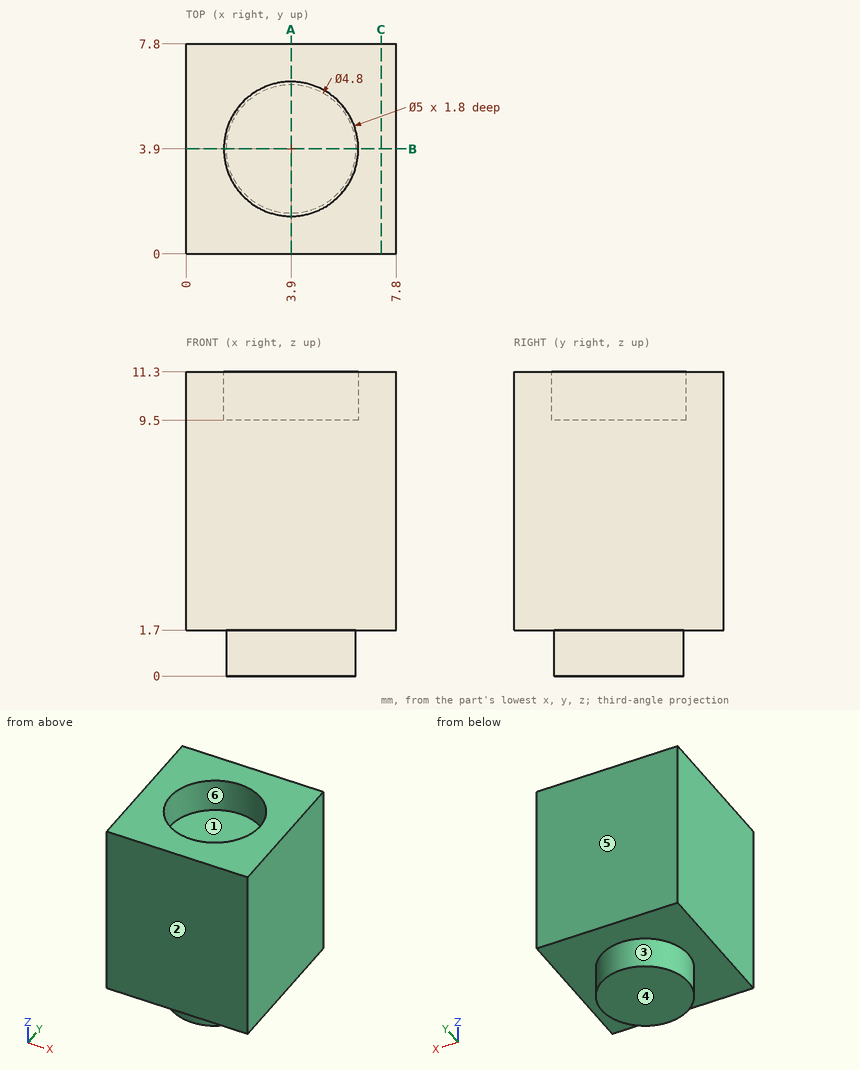
Geometry: see drawing. Coordinates: mm, zero at the bounding-box minimum. A direction names the side the tool comes from. Round coordinates to 2 decimals unless told otherwise and drop trailing zeros. Loops run counter-clockwise (first coordinate to the right, second up) from the corner with the lowest first, then second, coordinate; pieces in that order, holes last. Notation, with made-up numbers: (79, 83.25) -> (104, 83.25) arc R11 cw to (104, 104.25) -> close; hole circle Ø3 at (39.5, -18). An arc over 180 degrees is marked (long way). One line per question, with ' | ' between items. Start each with the question number.
1. Section C-C on x = 7.25. Output: boundary loops of the cut face in (y, z), and give its area (3 significant figures).
2. Line query: line 1 along Y through (x, z) = (3.9, 10.65); line 2 along Z through (x, y) = (5.5, 4.5); line 3 along Z through (x, y) = (4, 7.75). Output: solid intervals per line, ascending. Write a range as [from, to].
3. Mould query, pull axis Y, two halves, no side actions, for the marked faces 4, 5 and 6. Classes: pulls with the +Y half, pulls with the -Y half, needs draft (parallel to the pull), parting line crosses it, or undercut.
4. Section A-A on x = 3.9. Output: boundary loops of the cut face in (y, z), and give its area (3 significant figures).
5. Set-up query: the marked faces 1, 2 and 3. Return all of +Z, -Z, +X, -X, +Y, -Y with unobstructed straight access to the full face (end or side cutting, diameter ignored); none if empty.
6. Contact query for a flat-ended pin moving along its axis: pin 1 (3 mm diameter, centred on x = 3, y = 4, fed in from +Z). Output: stop coordinate, or through.
Returned:
1) outline: (0, 1.7) -> (7.8, 1.7) -> (7.8, 11.3) -> (0, 11.3) -> close | area: 74.9 mm2
2) line 1: y = [0, 1.4], [6.4, 7.8] | line 2: z = [0, 9.5] | line 3: z = [1.7, 11.3]
3) face 4: needs draft | face 5: pulls with the +Y half | face 6: undercut
4) outline: (0, 1.7) -> (1.5, 1.7) -> (1.5, 0) -> (6.3, 0) -> (6.3, 1.7) -> (7.8, 1.7) -> (7.8, 11.3) -> (6.4, 11.3) -> (6.4, 9.5) -> (1.4, 9.5) -> (1.4, 11.3) -> (0, 11.3) -> close | area: 74.0 mm2
5) face 1: +Z | face 2: +Z, -Z, +X, -X, -Y | face 3: -Z
6) pin 1: stops at z = 9.5
